Build history of the part. All positions in model axes, mm. A direction names the side the tool comes from. Round coordinates to 2 decimals unless told otherwise and drop trailing zeros. Order: outer loops, then holes, each group sorted by start corner. A loop starts at its lowest first (then second) coordinate and runs counter-clockwise, first axis right, second up. Notation, with made-up numbers: (87, 34.25) -> (100, 34.25) arc R20 cw to (100, 57.25) -> close; hole circle Ø4 at (-33, 29.5). An arc over 180 degrees is marked (long way). Use a Markdown table: item, result. Add a question column.
Item 1: Probe L1, parallel to Z at x = 0, y = -33; L2, parallel to Z at x = -1, y = -13; L3, parallel to X at y = -11.5, z = -3. List the from-to ranges inside material, lowest first.
Item 2: Slice it at C-C, the plane y = -8.5. Give the cut face in (x, z), plus the area to 3 significant figures.
Item 3: Slice it at B-B, the plane y = -14. Give the cut face in (x, z), plus the area to 3 significant figures.
Item 4: 3-axis set-ups, long thin cutter, end or side, ignore diameter. For faces 1 (the face through (2, 0, -3)), 2 (the face through (-2, -11.14, -5)), 3 (the face through (4.69, -3.52, -1.95)): which of +Z, -Z, +X, -X, +Y, -Y reach the whole face in a straight line?
Item 5: Pin check, flat tips, straight feed: pin 1 (5 mm diameter, centred on y = -28, z = 0, fed in from +X); pin 2 (5 mm diameter, centred on x = -0.5, y = -7, fed in from -Z); pin 3 (4 mm diameter, centred on x = 5.5, y = -9.5, fed in from -Z); pin 4 (5 mm diameter, centred on x = 2, z = -5, fed in from -Y). Stop position of each tip, or through.
Item 6: Two-plate mould, pull along X, no slides. Class faces 4 (the face through (3.05, -22.54, -1.26)), 5 (the face through (3.17, -6.57, -4.13)), 6 (the face through (1.1, -45.72, -3.3)): released by +X, released by -X, zero draft, split by the parting line, or undercut.
Item 7: Slice it at A-A, the plane x = 0. Give the cut face in (y, z), plus the area to 3 significant figures.
from build123d import *

# Parameters (mm, degrees)
F0_R     = 5.08
F0_R_2   = 3.302
F1_DEPTH = 45.72
F4_R     = 0.762


with BuildPart() as f1:
    # F0 (on Front) → F1 (new body)
    with BuildSketch(Plane.XZ):
        Circle(F0_R)
        Circle(F0_R_2, mode=Mode.SUBTRACT)
    extrude(amount=F1_DEPTH)

    # F2 (on Right) → F3 (revolve)
    with BuildSketch(Plane.YZ):
        Polygon((-11.139527, 7.112), (-11.139527, 5.08), (-6.35, 5.08), (-9.869527, 7.112), align=None)
    revolve(axis=Axis((0, -45.72, 0), (0, -1, 0)))

    # F4
    f4_edges = [f1.edges().sort_by_distance(p)[0] for p in [
        (-5.08, 0, 0),
    ]]
    fillet(f4_edges, radius=F4_R)


solid = f1.part
Check sheet entries:
| question | item | result |
|---|---|---|
| 1 | L1 | -5.08 to -3.3, 3.3 to 5.08 |
| 1 | L2 | -4.98 to -3.15, 3.15 to 4.98 |
| 1 | L3 | -4.1 to -1.38, 1.38 to 4.1 |
| 2 | outline | circle Ø12.64 at (0, 0); hole circle Ø6.6 at (0, 0) |
| 2 | area | 91.3 mm2 |
| 3 | outline | circle Ø10.16 at (0, 0); hole circle Ø6.6 at (0, 0) |
| 3 | area | 46.8 mm2 |
| 4 | face 1 | +Z, -Z, +X, -X, +Y |
| 4 | face 2 | -Y |
| 4 | face 3 | +Y |
| 5 | pin 1 | x = 5.08 |
| 5 | pin 2 | z = -6.89 |
| 5 | pin 3 | z = -6.17 |
| 5 | pin 4 | y = -45.72 |
| 6 | face 4 | undercut |
| 6 | face 5 | split by the parting line |
| 6 | face 6 | zero draft |
| 7 | outline | (-45.72, -5.08) -> (-11.14, -5.08) -> (-11.14, -7.11) -> (-9.87, -7.11) -> (-6.35, -5.08) -> (-0.76, -5.08) arc R0.76 ccw to (0, -4.32) -> (0, -3.3) -> (-45.72, -3.3) -> close; (-45.72, 3.3) -> (0, 3.3) -> (0, 4.32) arc R0.76 ccw to (-0.76, 5.08) -> (-6.35, 5.08) -> (-9.87, 7.11) -> (-11.14, 7.11) -> (-11.14, 5.08) -> (-45.72, 5.08) -> close |
| 7 | area | 175 mm2 |
